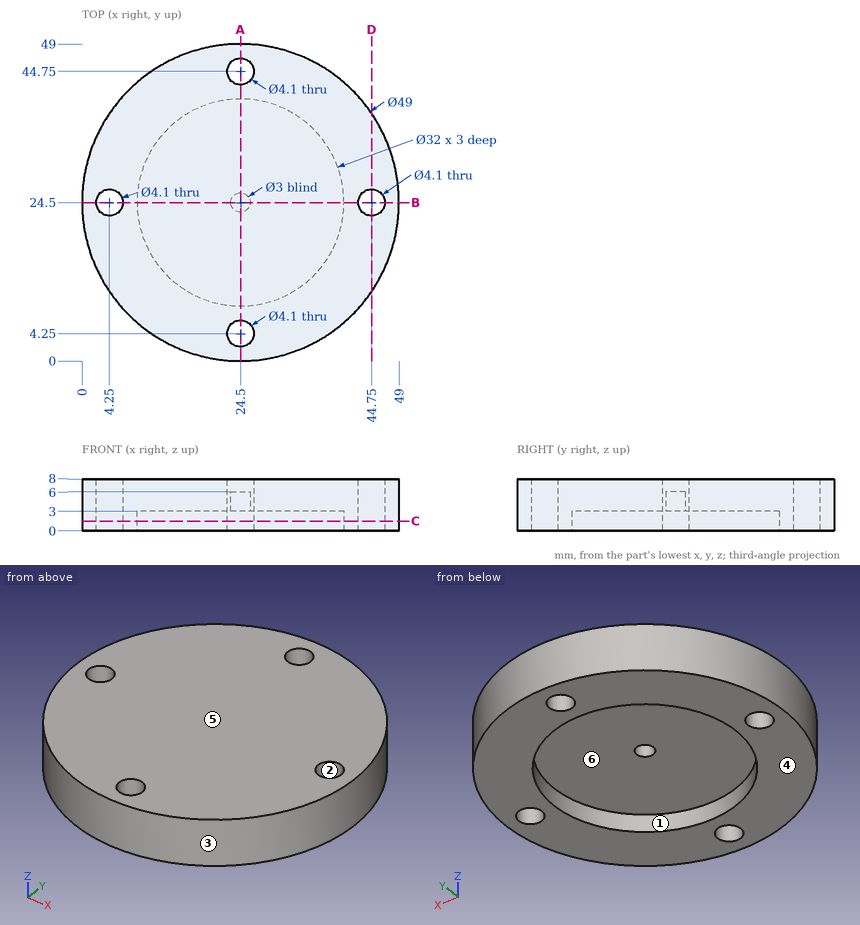
Part print with two shaded views. Sizes in mm from the minimum x, y, z corner. A direction names the side the tool comes from. Coordinates: 2 decimals unless noted, no trailing zeros. Write each loop counter-clockwise with the first axis right and the second up, starting at its lowest first coordinate (ties: lowest second). Pieces come first, ordered by that corner, then holes. Notation, with made-up numbers: (15.5, 64) - (28.5, 64) arc R13 cw to (28.5, 82) - close; hole circle Ø5 at (-37, 15.5). An arc over 180 degrees is marked (long way). Use a Markdown table: item, result. Add a question column.
Item 1: Drill centre lines: line 1 along Y through (x, z) = (24.5, 6.25); line 2 along Y through (x, z) = (24.5, 5.75); line 3 along X through (y, z) = (3.5, 5). Where is each one in solid material? Low to high.
Item 2: Two-plate mould, pull along X, no slides. Class the marked faces 1, 2, 3 and 4: pulls with the +X half, pulls with the -X half, needs draft (parallel to the pull), parting line crosses it, or undercut.
Item 3: 3-axis set-ups, long thin cutter, end or side, ignore diameter. For the marked faces 5 and 6: which of +Z, -Z, +X, -X, +Y, -Y reach the whole face in a straight line?
Item 4: Band-saw the part on C-C, the plane z = 1.5. Write the cut outline in (x, y), and give its area (3 significant figures).
Item 5: Band-saw the part on D-D, the plane x = 44.75. Write the cut outline in (y, z), and give its area (3 significant figures).
Item 6: Band-saw the part on A-A, the plane x = 24.5. Write the cut outline in (y, z), and give its area (3 significant figures).
Item 7: Drop flat-ended pins along their axis: pin 1 (1 mm diameter, centred on y = 32.5, z = 1, fed in from +X); pin 2 (1.5 mm diameter, centred on y = 8, z = 5.5, fed in from +X); pin 3 (1.5 mm diameter, centred on x = 24, y = 24, fed in from -Z); pin 4 (2.5 mm diameter, centred on x = 44.75, y = 24.5, fed in from +Z). Give the stop position or say it passes through.
A:
| question | item | result |
|---|---|---|
| 1 | line 1 | y = 0 to 2.2, 6.3 to 42.7, 46.8 to 49 |
| 1 | line 2 | y = 0 to 2.2, 6.3 to 23, 26 to 42.7, 46.8 to 49 |
| 1 | line 3 | x = 11.88 to 22.59, 26.41 to 37.12 |
| 2 | face 1 | undercut |
| 2 | face 2 | undercut |
| 2 | face 3 | parting line crosses it |
| 2 | face 4 | needs draft |
| 3 | face 5 | +Z, +X, -X, +Y, -Y |
| 3 | face 6 | -Z |
| 4 | outline | circle Ø49 at (24.5, 24.5); hole circle Ø4.1 at (4.25, 24.5); hole circle Ø32 at (24.5, 24.5); hole circle Ø4.1 at (24.5, 4.25); hole circle Ø4.1 at (24.5, 44.75); hole circle Ø4.1 at (44.75, 24.5) |
| 4 | area | 1,030 mm² |
| 5 | outline | (10.71, 0) - (22.45, 0) - (22.45, 8) - (10.71, 8) - close; (26.55, 0) - (38.29, 0) - (38.29, 8) - (26.55, 8) - close |
| 5 | area | 188 mm² |
| 6 | outline | (0, 0) - (2.2, 0) - (2.2, 8) - (0, 8) - close; (6.3, 0) - (8.5, 0) - (8.5, 3) - (23, 3) - (23, 6) - (26, 6) - (26, 3) - (40.5, 3) - (40.5, 0) - (42.7, 0) - (42.7, 8) - (6.3, 8) - close; (46.8, 0) - (49, 0) - (49, 8) - (46.8, 8) - close |
| 6 | area | 221 mm² |
| 7 | pin 1 | stops at x = 47.82 |
| 7 | pin 2 | stops at x = 43.27 |
| 7 | pin 3 | stops at z = 6 |
| 7 | pin 4 | passes through |
